Here's how the part is built. I have some questions about the finished solid (model axes, mm). Round coordinates to 2 decimals unless told otherwise and drop trailing zeros. Order: outer loops, then holes, each group sorted by start corner. A loop starts at its lowest first (then second) coordinate and runs counter-clockwise, first axis right, second up. Notation, with made-up numbers: (-7.75, -4.75) -> (31.25, -4.75) arc R12 ccw to (31.25, 15.25) -> close; hole circle Ø5 at (-14.5, -36). An arc over 180 degrees is marked (long way). Answer in a Markdown table with one row per item.
```python
from build123d import *

# Parameters (mm, degrees)
SKETCH2_W           = 96
SKETCH2_H           = 96
BOSS_EXTRUDE1_DEPTH = 1.6
SKETCH3_R           = 1.55
SKETCH3_R_2         = 1.505
CUT_EXTRUDE1_DEPTH  = 2.6
SKETCH4_OUTSIDE_W   = 125.154
SKETCH4_OUTSIDE_H   = 125.154
SKETCH4_OUTSIDE_W_2 = 80
SKETCH4_OUTSIDE_H_2 = 80
CUT_EXTRUDE2_DEPTH  = 10


with BuildPart() as part:
    # Sketch2 → Boss-Extrude1 (new body)
    with BuildSketch(Plane(origin=(0, 0, 0), x_dir=(1, 0, 0), z_dir=(0, 1, 0))):
        with Locations((48, 48)):
            Rectangle(SKETCH2_W, SKETCH2_H)
    extrude(amount=BOSS_EXTRUDE1_DEPTH)

    # Sketch3 → Cut-Extrude1 (cut, through all)
    with BuildSketch(Plane(origin=(0, 1.6, 0), x_dir=(1, 0, 0), z_dir=(0, 1, 0))):
        with Locations((24, 48)):
            Circle(SKETCH3_R)
        with Locations((72, 48)):
            Circle(SKETCH3_R)
        with Locations((48, 72)):
            Circle(SKETCH3_R_2)
        with Locations((48, 24)):
            Circle(SKETCH3_R_2)
        with Locations((18, 78)):
            Circle(SKETCH3_R_2)
        with Locations((78, 78)):
            Circle(SKETCH3_R_2)
        with Locations((78, 18)):
            Circle(SKETCH3_R_2)
        with Locations((18, 18)):
            Circle(SKETCH3_R_2)
    extrude(amount=-CUT_EXTRUDE1_DEPTH, mode=Mode.SUBTRACT)

    # Sketch4 outside → Cut-Extrude2 (cut)
    with BuildSketch(Plane(origin=(0, 1.6, 0), x_dir=(1, 0, 0), z_dir=(0, 1, 0))):
        with Locations((48, 48)):
            Rectangle(SKETCH4_OUTSIDE_W, SKETCH4_OUTSIDE_H)
        with Locations((48, 48)):
            Rectangle(SKETCH4_OUTSIDE_W_2, SKETCH4_OUTSIDE_H_2, mode=Mode.SUBTRACT)
    extrude(amount=-CUT_EXTRUDE2_DEPTH, mode=Mode.SUBTRACT)


solid = part.part
```
1. We'd pull the mould along Z, two halves only. Please class faces 1 (the face through (79.436, 0.811, -78.452)), 2 (the face through (47, 1.6, -49)), 3 (the face through (18.81, 0.81, -19.27)): released by +Z, released by -Z, zero draft, split by the parting line, or undercut.
Numbers:
| item | result |
|---|---|
| face 1 | undercut |
| face 2 | zero draft |
| face 3 | undercut |
2. Suppose I cut it at B-B on z = -24. Write out the boundary of the cut face in (x, y) (3 decimals), then the cut area to 3 significant figures.
Numbers:
| item | result |
|---|---|
| outline | (8, 0) -> (46.495, 0) -> (46.495, 1.6) -> (8, 1.6) -> close; (49.505, 0) -> (88, 0) -> (88, 1.6) -> (49.505, 1.6) -> close |
| area | 123 mm2 |
3. Suppose I cut it at C-C on z = -78. Write out the boundary of the cut face in (x, y) (3 decimals).
Numbers:
| item | result |
|---|---|
| outline | (8, 0) -> (16.495, 0) -> (16.495, 1.6) -> (8, 1.6) -> close; (19.505, 0) -> (76.495, 0) -> (76.495, 1.6) -> (19.505, 1.6) -> close; (79.505, 0) -> (88, 0) -> (88, 1.6) -> (79.505, 1.6) -> close |
4. Please list where these lines run through material, in increasing order: line 1 along Z through (x, y) = (78, 1) (3 decimals); line 2 along X through (y, z) = (1, -18) (3 decimals); line 3 along Z through (x, y) = (48, 0.7) (3 decimals).
Numbers:
| item | result |
|---|---|
| line 1 | z = -88 to -79.505, -76.495 to -19.505, -16.495 to -8 |
| line 2 | x = 8 to 16.495, 19.505 to 76.495, 79.505 to 88 |
| line 3 | z = -88 to -73.505, -70.495 to -25.505, -22.495 to -8 |
5. For pin 1 Ø2.5 at (x, z) = (72, -48) entering from +Y, with a flat end and sliding along its axis, tell me the tip position at first contact or that it passes through.
Numbers:
| item | result |
|---|---|
| pin 1 | passes through |
6. Suppose I cut it at A-A on x = 18. Write out the boundary of the cut face in (y, z) (3 decimals).
Numbers:
| item | result |
|---|---|
| outline | (0, -88) -> (1.6, -88) -> (1.6, -79.505) -> (0, -79.505) -> close; (0, -76.495) -> (1.6, -76.495) -> (1.6, -19.505) -> (0, -19.505) -> close; (0, -16.495) -> (1.6, -16.495) -> (1.6, -8) -> (0, -8) -> close |
